Design review of the part shown in the three views and the two pictorial views. Dimensions are in mm from the part's minimum x, y and z. A direction names the side the tool comes from. Coordinates: 2 decimals unless noted, no trailing zeros. Loops run counter-clockwise (first coordinate to the right, second up) from the corner with the lowest first, then second, coordinate; pieces in that order, holes last. Notation, with made-up numbers: (36.5, 86) -> (45.5, 86) arc R20 cw to (45.5, 119) -> close; hole circle Ø6 at (-23.5, 77.5). An arc over 180 degrees is marked (long way). One line per item, written item: value.
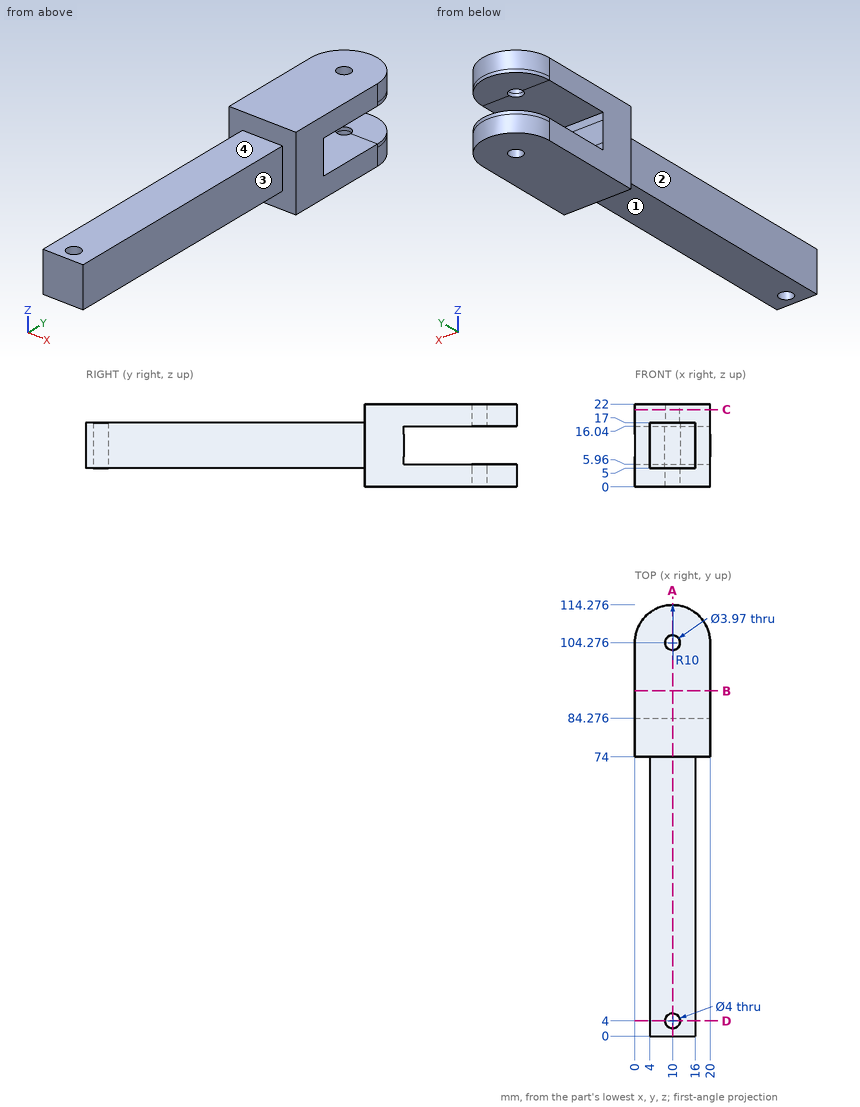
1. Insertion check: pin 1 Ø6.5 at (x, z) = (13, 12) entering from +Y; pin 2 Ø1 at (x, y) = (13, 52) entering from -Z; pin 3 Ø8 at (x, y) = (2, 30.5) entering from +Z; pin 4 Ø4.5 at (x, y) = (10, 104.28) entering from +Z. Each pin has a flat end and moves straight along its axis. Give the tip position at first contact, or say it passes through.
Return value:
pin 1: stops at y = 84.28
pin 2: stops at z = 5
pin 3: stops at z = 17
pin 4: stops at z = 22
2. To check wall thickness, follow probe 1 along Y at (x, z) = (10, 5.4); probe 2 along Y at (x, z) = (8.75, 16.75) (1 decimal); probe 3 along Z at (x, y) = (16.25, 95). State the ranges of each line that lie inside material, in increasing order. Write a range as from..to.
Return value:
probe 1: y = 0..2, 6..102.29, 106.26..114.28
probe 2: y = 0..2.4, 5.6..102.7, 105.8..114.2
probe 3: z = 0..5.96, 16.04..22
3. Take a section at D-D, the plane y = 4. Give the boundary of the cut face in (x, z).
Return value:
outline: (4, 5) -> (8, 5) -> (8, 17) -> (4, 17) -> close; (12, 5) -> (16, 5) -> (16, 17) -> (12, 17) -> close
4. Take a section at C-C, the plane z = 20.5. Give the boundary of the cut face in (x, y) (1 decimal).
Return value:
outline: (0, 74) -> (20, 74) -> (20, 104.3) arc R10 ccw to (0, 104.3) -> close; hole circle Ø4 at (10, 104.3)
5. Take a section at B-B, the plane y = 91.5. Give the boundary of the cut face in (x, z), and give its area (3 significant figures).
Return value:
outline: (0, 0) -> (20, 0) -> (20, 5.96) -> (0, 5.96) -> close; (0, 16.04) -> (20, 16.04) -> (20, 22) -> (0, 22) -> close
area: 238 mm2
6. For the marked faces 1, 2, 3 and 4, list the 3-axis set-ups (+Z, -Z, +X, -X, +Y, -Y) from which the entire face can be reached by the end or side of a thin tool; tool diameter is ignored.
Return value:
face 1: -Z, +X, -X, -Y
face 2: +Z, -Z, -X, -Y
face 3: +Z, -Z, +X, -Y
face 4: +Z, +X, -X, -Y
7. Take a section at A-A, the plane x = 10. Give the boundary of the cut face in (y, z).
Return value:
outline: (0, 5) -> (2, 5) -> (2, 17) -> (0, 17) -> close; (6, 5) -> (74, 5) -> (74, 0) -> (102.29, 0) -> (102.29, 5.96) -> (84.28, 5.96) -> (84.28, 16.04) -> (102.29, 16.04) -> (102.29, 22) -> (74, 22) -> (74, 17) -> (6, 17) -> close; (106.26, 0) -> (114.28, 0) -> (114.28, 5.96) -> (106.26, 5.96) -> close; (106.26, 16.04) -> (114.28, 16.04) -> (114.28, 22) -> (106.26, 22) -> close
